Geometry check sheet. Reference: drawing and pictorial views, mm from the part's lowest x, y, z. A direction names the side the tool comes from. Round coordinates to 2 decimals unless told otherwise and drop trailing zeros. Order: outer loops, then holes, each group sorted by start corner. A loop starts at its lowest first (then second) coordinate and runs counter-clockwise, first axis right, second up.
(1) Cross-section at A-A on x = 5. Enter the section's corners in (y, z).
(2) Thickness scan on L1, parallel to Z at x = 5, y = 4.25; L2, parallel to Y at x = 2, z = 7.25; L3, parallel to X at y = 8, z = 4. Record the ranges inside material, lowest first.
(3) Gauge pin test, flat ends, axial feed: P1, Ø6, axis at x = 5, z = 5, coming from the +Y side; P2, Ø5, axis at x = 5, y = 4.5, coming from the -Z side; P3, Ø1, axis at x = 9, z = 8.5, coming from the -Y side; P4, Ø4, axis at y = 7, z = 6, coming from the +X side. Record the tip position at first contact, or that the pin passes through.
(4) Cross-section at B-B on z = 5. Enter the section's corners in (x, y).
(5) Cross-section at D-D on x = 2. Enter the section's corners in (y, z).
(6) Set-up check for the marked faces 4 and 5: record each of +Z, -Z, +X, -X, +Y, -Y from which the full face is reachable in a straight line by a thin tool's end or side.
(7) Draft check along Z on the marked faces 1, 2 and 3. Enter one of: pulls with the +Z half, pulls with the -Z half, needs draft (parallel to the pull), parting line crosses it, or undercut.
(8) Cross-section at C-C on y = 6.75. Enter the section's corners in (x, z), and give its area (3 significant figures).
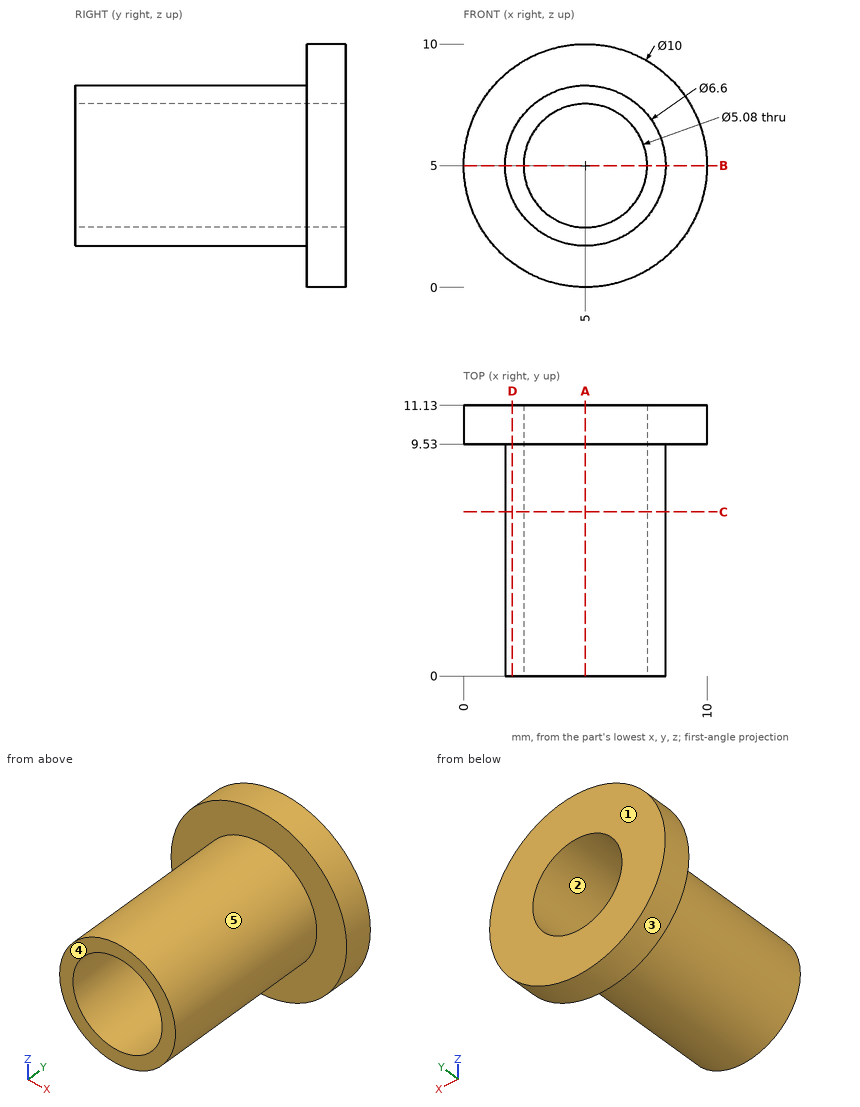
Found:
1. outline: (0, 1.7) - (9.53, 1.7) - (9.53, 0) - (11.13, 0) - (11.13, 2.46) - (0, 2.46) - close; (0, 7.54) - (11.13, 7.54) - (11.13, 10) - (9.53, 10) - (9.53, 8.3) - (0, 8.3) - close
2. L1: z = 1.7 to 2.46, 7.54 to 8.3
2. L2: y = 9.53 to 11.13
2. L3: x = 1.86 to 2.67, 7.33 to 8.14
3. P1: stops at y = 11.13
3. P2: stops at z = 1.7
3. P3: stops at y = 9.53
3. P4: stops at x = 8.3
4. outline: (0, 9.53) - (1.7, 9.53) - (1.7, 0) - (2.46, 0) - (2.46, 11.13) - (0, 11.13) - close; (7.54, 0) - (8.3, 0) - (8.3, 9.53) - (10, 9.53) - (10, 11.13) - (7.54, 11.13) - close
5. outline: (0, 3.63) - (9.53, 3.63) - (9.53, 1) - (11.13, 1) - (11.13, 9) - (9.53, 9) - (9.53, 6.37) - (0, 6.37) - close
6. face 4: +Z, -Z, +X, -X, -Y
6. face 5: -Y
7. face 1: needs draft
7. face 2: undercut
7. face 3: parting line crosses it
8. outline: circle Ø6.6 at (5, 5); hole circle Ø5.08 at (5, 5)
8. area: 13.9 mm2
